```python
from build123d import *

# Parameters (mm, degrees)
SKETCH1_W                                     = 31.75
SKETCH1_H                                     = 6.35
BOSS_EXTRUDE1_DEPTH                           = 46.99
F_4_40_TAPPED_HOLE1_D                         = 2.2606
F_4_40_TAPPED_HOLE1_DEPTH                     = 7.5946
F_4_40_TAPPED_HOLE1_TIP                       = 0.679152758
CBORE_START                                   = 0.3302
CBORE_SLOT_FOR_4_SOCKET_HEAD_CAP_SCREW1_DEPTH = 2.8448
CBORE_START_2                                 = -3.175
CBORE_SLOT_FOR_4_SOCKET_HEAD_CAP_SC_3_DEPTH   = 3.5052


# Read off the part's stored shape, not the designer's step: CBORE SLOT for #4 Socket Head Cap Screw1
with BuildPart() as part:
    # Sketch1 → Boss-Extrude1 (new body)
    with BuildSketch(Plane(origin=(0, 0, 0), x_dir=(1, 0, 0), z_dir=(0, 1, 0))):
        Rectangle(SKETCH1_W, SKETCH1_H)
    extrude(amount=BOSS_EXTRUDE1_DEPTH)

    # #4-40 Tapped Hole1
    with Locations(Plane(origin=(0, 0, 0), x_dir=(-1, 0, 0), z_dir=(0, -1, 0))):
        with Locations((9.525, 0), (-9.525, 0)):
            Hole(F_4_40_TAPPED_HOLE1_D / 2, depth=F_4_40_TAPPED_HOLE1_DEPTH)
            with Locations((0, 0, -(F_4_40_TAPPED_HOLE1_DEPTH + F_4_40_TAPPED_HOLE1_TIP / 2))):  # 118° drill point
                Cone(0, F_4_40_TAPPED_HOLE1_D / 2, F_4_40_TAPPED_HOLE1_TIP, mode=Mode.SUBTRACT)

    # CBORE SLOT for _4 Socket Head Cap Sc 2 → CBORE SLOT for #4 Socket Head Cap Screw1 (cut)
    with BuildSketch(Plane.XY.offset(CBORE_START)):
        with BuildLine():
            Line((-6.74624, 40.36695), (-6.74624, 43.45305))
            ThreePointArc((-6.74624, 43.45305), (-9.525, 46.23181), (-12.30376, 43.45305))
            Line((-12.30376, 43.45305), (-12.30376, 40.36695))
            ThreePointArc((-12.30376, 40.36695), (-9.525, 37.58819), (-6.74624, 40.36695))
        make_face()
        with BuildLine():
            Line((12.30376, 40.36695), (12.30376, 43.45305))
            ThreePointArc((12.30376, 43.45305), (9.525, 46.23181), (6.74624, 43.45305))
            Line((6.74624, 43.45305), (6.74624, 40.36695))
            ThreePointArc((6.74624, 40.36695), (9.525, 37.58819), (12.30376, 40.36695))
        make_face()
    extrude(amount=CBORE_SLOT_FOR_4_SOCKET_HEAD_CAP_SCREW1_DEPTH, mode=Mode.SUBTRACT)

    # CBORE SLOT for _4 Socket Head Cap Sc 3 o → CBORE SLOT for _4 Socket Head Cap Sc 3 (cut)
    with BuildSketch(Plane.XY.offset(CBORE_START_2)):
        with BuildLine():
            ThreePointArc((-7.89305, 43.45305), (-9.525, 45.085), (-11.15695, 43.45305))
            Line((-11.15695, 43.45305), (-11.15695, 40.36695))
            ThreePointArc((-11.15695, 40.36695), (-9.525, 38.735), (-7.89305, 40.36695))
            Line((-7.89305, 40.36695), (-7.89305, 43.45305))
        make_face()
        with BuildLine():
            Line((7.89305, 43.45305), (7.89305, 40.36695))
            ThreePointArc((7.89305, 40.36695), (9.525, 38.735), (11.15695, 40.36695))
            Line((11.15695, 40.36695), (11.15695, 43.45305))
            ThreePointArc((11.15695, 43.45305), (9.525, 45.085), (7.89305, 43.45305))
        make_face()
    extrude(amount=CBORE_SLOT_FOR_4_SOCKET_HEAD_CAP_SC_3_DEPTH, mode=Mode.SUBTRACT)


solid = part.part
```
Model file for the job. Use its own axes, mm. A direction names the side the tool comes from. Coordinates: 2 decimals unless noted, no trailing zeros. Order: outer loops, then holes, each group sorted by start corner. A loop starts at its lowest first (then second) coordinate and runs counter-clockwise, first axis right, second up. Notation, with made-up numbers: (4, -19) - (25, -19) arc R24 cw to (25, 10) - close; hole circle Ø3 at (42.5, -3). An arc over 180 degrees is marked (long way). Return JSON: item names as keys, results as strings. Group by question number.
1) Tool access for faces 1 (the cylindrical face through (10.57, 3.85, 0.43)), 2 (the cylindrical face through (-9.59, 37.59, 1.73)), 3 (the cylindrical face through (-9, 45, -1)), 4 (the flat face through (0, 23, 3.175)): list every direction of +Z, -Z, +X, -X, +Y, -Y with a clear straight run to the whole face (end or side of a thin tool).
2) Mould opens along Y. For faces 5 (the conical face through (9.434, 8.156, 0.174)), 6 (the cylindrical face through (-9.46, 46.23, 1.73)), 7 (the flat face through (0, 46.99, 0)), 8 (the cylindrical face through (-10.654, 3.85, -0.05)) say: released by +Y, released by -Y, zero draft, split by the parting line, or undercut.
3) Saw through at A-A, the plane y = 5.5. Write the cut outline in (x, z) (3 decimals).
4) Probe line 1 (X direction, y = 44.5, z = -1.25) (3 decimals); line 2 (Z direction, x = -7, y = 43.5) (3 decimals); line 3 (Y direction, x = 11, z = -0.25). List the from-to ranges inside material, lowest first. Write a range as from..to.
5) Flat gauge pins, fed straight in: P1, Ø2, axis at x = 9.525, z = 0, coming from the -Y side; P2, Ø1.7, axis at x = -10.5, y = 42.5, coming from the +Z side. Where does each tip first touch, or does it go through?
6) Saw through at B-B, the plane z = 2.25. Write the cut outline in (x, y) (3 decimals).
Values found:
{
 "1": {"face 1": "-Y", "face 2": "+Z", "face 3": "+Z, -Z", "face 4": "+Z, +X, -X, +Y, -Y"},
 "2": {"face 5": "released by -Y", "face 6": "undercut", "face 7": "released by +Y", "face 8": "zero draft"},
 "3": {"outline": "(-15.875, -3.175) - (15.875, -3.175) - (15.875, 3.175) - (-15.875, 3.175) - close; hole circle Ø2.261 at (-9.525, 0); hole circle Ø2.261 at (9.525, 0)"},
 "4": {"line 1": "x = -15.875..-10.777, -8.273..8.273, 10.777..15.875", "line 2": "z = -3.175..0.33", "line 3": "y = 0..39.67, 44.15..46.99"},
 "5": {"P1": "stops at y = 7.67", "P2": "stops at z = 0.33"},
 "6": {"outline": "(-15.875, 0) - (15.875, 0) - (15.875, 46.99) - (-15.875, 46.99) - close; hole (-12.304, 40.367) arc R2.779 ccw to (-6.746, 40.367) - (-6.746, 43.453) arc R2.779 ccw to (-12.304, 43.453) - close; hole (6.746, 40.367) arc R2.779 ccw to (12.304, 40.367) - (12.304, 43.453) arc R2.779 ccw to (6.746, 43.453) - close"}
}
